Source: CAD feature listing. Evaluate the final solid. Frame: model axes, mm. Round coordinates to 2 decimals unless told otherwise and drop trailing zeros. Loops run counter-clockwise (first coordinate to the right, second up) from the corner with the lowest first, then second, coordinate; pieces in that order, holes last.
Item 1: Pull-direction query (Y, two-part tool) for faces 1 (the flat face through (-60, 0, 15)), 2 (the cylindrical face through (-55, 0, 15)), 3 (the flat face through (-1, -17.5, 15)); classes: released by +Y, released by -Y, zero draft, split by the parting line, or undercut.
Item 2: Section query B-B on y = 0. Return loops of the section in (x, z).
Item 3: Section query A-A on x = -45. Return loops of the section in (y, z).
Item 4: Ray query, L1, parallel to Y at x = -45, z = 18.5; L2, parallel to X at y = -0.5, z = 25.75; L3, parallel to X at y = -1, z = 19. Return the intervals inside material, ascending.
Item 5: Section query C-C on z = 19.25. Return loops of the section in (x, y), then the cut area to 3 significant figures.
```python
from build123d import *

# Parameters (mm, degrees)
F0_W      = 120
F0_H      = 35
F0_R      = 10
F1_DEPTH  = 5
F1_FACE_W = 120
F1_FACE_H = 35
F1_FACE_R = 10
F2_DEPTH  = 25


with BuildPart() as f1:
    # F0 (on Top) → F1 (new body)
    with BuildSketch(Plane.XY):
        Rectangle(F0_W, F0_H)
        with Locations((-45, 0)):
            Circle(F0_R, mode=Mode.SUBTRACT)
    extrude(amount=F1_DEPTH)

    # F1_face (on face) → F2 (join)
    with BuildSketch(Plane(origin=(3.638123, 0, 5), x_dir=(1, 0, 0), z_dir=(0, 0, 1))):
        with Locations((-3.638123, 0)):
            Rectangle(F1_FACE_W, F1_FACE_H)
        with Locations((-48.638123, 0)):
            Circle(F1_FACE_R, mode=Mode.SUBTRACT)
    extrude(amount=F2_DEPTH)


solid = f1.part
```
Data:
1. face 1: zero draft
1. face 2: undercut
1. face 3: released by -Y
2. outline: (-60, 0) - (-55, 0) - (-55, 30) - (-60, 30) - close; (-35, 0) - (60, 0) - (60, 30) - (-35, 30) - close
3. outline: (-17.5, 0) - (-10, 0) - (-10, 30) - (-17.5, 30) - close; (10, 0) - (17.5, 0) - (17.5, 30) - (10, 30) - close
4. L1: y = -17.5 to -10, 10 to 17.5
4. L2: x = -60 to -54.99, -35.01 to 60
4. L3: x = -60 to -54.95, -35.05 to 60
5. outline: (-60, -17.5) - (60, -17.5) - (60, 17.5) - (-60, 17.5) - close; hole circle Ø20 at (-45, 0)
5. area: 3,890 mm2
